Source: CAD feature listing. Evaluate the final solid. Frame: model axes, mm. A direction names the side the tool comes from. Give positions to 0.01 mm unless a question says otherwise; leave off trailing zeros. Write each loop counter-clockwise with the first axis right and the second up, starting at its lowest first coordinate (ties: lowest second). Pieces come first, ordered by that corner, then holes. Notation, with made-up numbers: (40.5, 9) -> (73.5, 9) arc R14 ccw to (73.5, 24) -> close; hole circle Ø6 at (84, 2). An arc over 180 degrees is marked (long way). Write item = value, one per line.
from build123d import *

# Parameters (mm, degrees)
F1_DEPTH = 7.5
F2_DEPTH = 4.5
F3_R     = 2.3
F4_DEPTH = 5
F5_SIZE  = 1.8
F6_R     = 1.99999


# Not quite as in the source:
# - a fillet or chamfer is up to 0.001 mm smaller than in the source, because OpenCascade refuses the exact size


with BuildPart() as f1:
    # F0 (on Front) → F1 (new body, symmetric)
    with BuildSketch(Plane.XZ):
        Polygon((2, 16), (0, 16), (0, 0), (2, 0), (2, -7.7), (5.15, -7.7), (5.15, -5.7), (4, -5.7), (4, 0), (28, 0), (28, -5.7), (26.85, -5.7), (26.85, -7.7), (30, -7.7), (30, 2), (14, 2), (2, 2), (2, 7.5), align=None)
        Polygon((14, 2), (2, 7.5), (2, 2), align=None)
    extrude(amount=F1_DEPTH, both=True)

    # F0 (on Front) → F2 (cut, symmetric)
    with BuildSketch(Plane.XZ):
        Polygon((14, 2), (2, 7.5), (2, 2), align=None)
    extrude(amount=F2_DEPTH, both=True, mode=Mode.SUBTRACT)

    # F3 (on face) → F4 (cut)
    with BuildSketch(Plane(origin=(0, 0, 0), x_dir=(0, -1, 0), z_dir=(-1, 0, 0))):
        with Locations((0, 8)):
            Circle(F3_R)
    extrude(amount=-F4_DEPTH, mode=Mode.SUBTRACT)

    # F5
    f5_edges = [f1.edges().sort_by_distance(p)[0] for p in [
        (2, 2.3, 8),
    ]]
    chamfer(f5_edges, length=F5_SIZE)

    # F6 (radius 2 in the source; OpenCascade refuses exactly that, so slightly less here)
    f6_edges = [f1.edges().sort_by_distance(p)[0] for p in [
        (2, -6, 7.5),
        (14, 6, 2),
        (14, -6, 2),
        (2, 6, 7.5),
        (2, 0, 0),
    ]]
    fillet(f6_edges, radius=F6_R)


solid = f1.part
(1) Material intervals for line 1 (X direction, y = -1.75, z = -4.5); line 2 (Z direction, x = 0.1, y = 0); line 3 (X direction, y = -2.25, z = -6.25), sorted ascending.
Values follow:
line_1 = 2 to 4, 28 to 30
line_2 = 0 to 5.7, 10.3 to 16
line_3 = 2 to 5.15, 26.85 to 30
(2) Access query for faces 4 (the face through (4, 0, -3)), 5 (the face through (2, -2, 12)), 6 (the face through (5.15, 0, -7)). Directions: +Z, -Z, +X, -X, +Y, -Y. A direction counts if a zero-diameter tool reaches every point of the face in a straight line with its end or side. Return the directions, or none.
Values follow:
face_4 = +Y, -Y
face_5 = +Z, +X
face_6 = -Z, +Y, -Y
(3) First-contact query: pin 1 (1.5 mm diameter, centred on x = 13.5, y = -2.5, fed in from +Z); pin 2 (6 mm diameter, centred on x = 10.5, y = 1.5, fed in from -Z); pin 3 (6.5 mm diameter, centred on y = 2, z = -5.5, fed in from -X). Flat tips, straight axial feed; report the tip coordinate or a pass-through.
Values follow:
pin_1 = 2
pin_2 = 0
pin_3 = 2
(4) Section query A-A (z = -2.75). Return loops of the section in (x, y), plus the area to 3 significant figures.
Values follow:
outline = (2, -7.5) -> (4, -7.5) -> (4, 7.5) -> (2, 7.5) -> close; (28, -7.5) -> (30, -7.5) -> (30, 7.5) -> (28, 7.5) -> close
area = 60.0 mm2
(5) Section query D-D (z = 3.5). Return loops of the section in (x, y), plus the area to 3 significant figures.
Values follow:
outline = (0, -7.5) -> (10.73, -7.5) -> (10.73, -4.5) -> (2, -4.5) -> (2, 4.5) -> (10.73, 4.5) -> (10.73, 7.5) -> (0, 7.5) -> close
area = 82.4 mm2
(6) Pull-direction query (X, two-part tool) for faces 1 (the face through (26.85, 0, -7)), 2 (the face through (1, 0, 16)), 3 (the face through (30, 0, -3)); classes: pulls with the +X half, pulls with the -X half, needs draft (parallel to the pull), parting line crosses it, or undercut.
Values follow:
face_1 = undercut
face_2 = needs draft
face_3 = pulls with the +X half
